Could you check a few things on this drawing? It's one solid part, dimensions in mm from its lowest x, y, z. A direction names the side the tool comes from. Coordinates: 2 decimals unless noted, no trailing zeros. Order: outer loops, then holes, each group sorted by start corner. A loop starts at its lowest first (then second) coordinate and runs counter-clockwise, first axis right, second up. Notation, with made-up numbers: (-39.5, -7) -> (11.5, -7) arc R27 cw to (11.5, 25) -> close; hole circle Ø7 at (59.5, 84.5). An arc over 180 degrees is marked (long way). Use a Markdown table: item, result. Add a question column.
1. For pin 1 Ø2.5 at (x, y) = (6.5, 6.5) entering from -Z (3 decimals); pin 2 Ø1 at (x, z) = (10.5, 1) entering from -Y; pin 3 Ø2 at (x, z) = (10.5, 5.5) entering from +Y, each with a flat end and sliding along its axis, tell me the tip position at first contact or that it passes through.
2. We'd pull the mould along Z, two halves only. Please class the marked faces 1, 2, 3 and 4: pulls with the +Z half, pulls with the -Z half, needs draft (parallel to the pull), parting line crosses it, or undercut.
3. Suppose I cut it at A-A, the plane x = 6.5. List the corners of the cut face in (y, z) for me.
4. For the marked faces 5 and 6, which set-ups out of +Z, -Z, +X, -X, +Y, -Y let a thin tool reach every point of the face, with its end or its side?
5. Suppose I cut it at D-D, the plane x = 10.25. List the corners of the cut face in (y, z) for me, then the cut area to 3 significant figures.
6. Suppose I cut it at C-C, the plane z = 5. List the corners of the cut face in (x, y) for me.
7. If I drill on line 1 along Z through (x, y) = (9.5, 2.25); line 2 along Y through (x, z) = (6.5, 0.7); line 3 along Y through (x, z) = (6.5, 2.35), over which ranges is the centre line in solid material (lowest first)? Write a range as from..to.
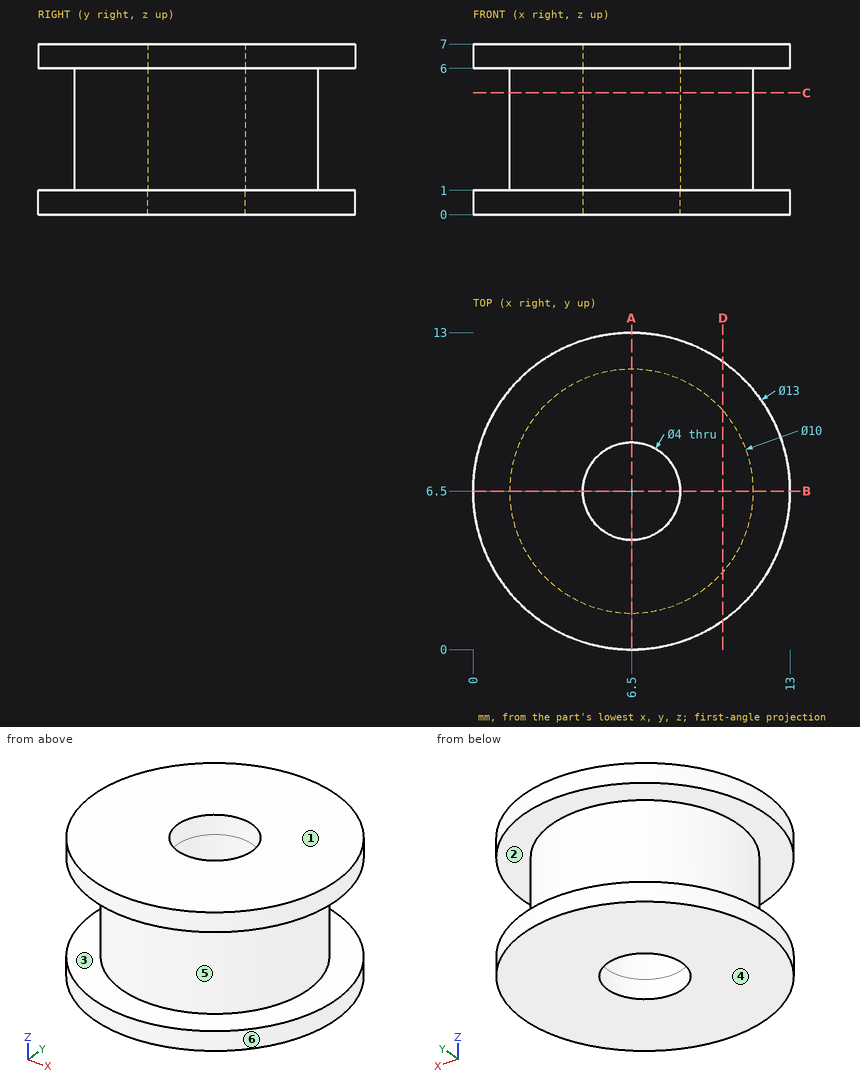
Worked out:
| question | item | result |
|---|---|---|
| 1 | pin 1 | passes through |
| 1 | pin 2 | stops at y = 1.02 |
| 1 | pin 3 | stops at y = 12.19 |
| 2 | face 1 | pulls with the +Z half |
| 2 | face 2 | undercut |
| 2 | face 3 | undercut |
| 2 | face 4 | pulls with the -Z half |
| 3 | outline | (0, 0) -> (4.5, 0) -> (4.5, 7) -> (0, 7) -> (0, 6) -> (1.5, 6) -> (1.5, 1) -> (0, 1) -> close; (8.5, 0) -> (13, 0) -> (13, 1) -> (11.5, 1) -> (11.5, 6) -> (13, 6) -> (13, 7) -> (8.5, 7) -> close |
| 4 | face 5 | none |
| 4 | face 6 | +Z, -Z |
| 5 | outline | (1.19, 0) -> (11.81, 0) -> (11.81, 1) -> (9.81, 1) -> (9.81, 6) -> (11.81, 6) -> (11.81, 7) -> (1.19, 7) -> (1.19, 6) -> (3.19, 6) -> (3.19, 1) -> (1.19, 1) -> close |
| 5 | area | 54.3 mm² |
| 6 | outline | circle Ø10 at (6.5, 6.5); hole circle Ø4 at (6.5, 6.5) |
| 7 | line 1 | z = 0..1, 6..7 |
| 7 | line 2 | y = 0..4.5, 8.5..13 |
| 7 | line 3 | y = 1.5..4.5, 8.5..11.5 |
